The drawing under review shows one solid part. Ordinate dimensions are in mm from its lowest x, y, z. A direction names the side the tool comes from. Coordinates: 2 decimals unless noted, no trailing zeros. Loops run counter-clockwise (first coordinate to the right, second up) from the corner with the lowest first, then second, coordinate; pieces in that order, holes last. Notation, with made-up numbers: (-22, 76) -> (13, 76) arc R38 ccw to (13, 114) -> close; hole circle Ø8 at (21.5, 3). An arc over 180 degrees is marked (long way). Use a Markdown table: item, result.
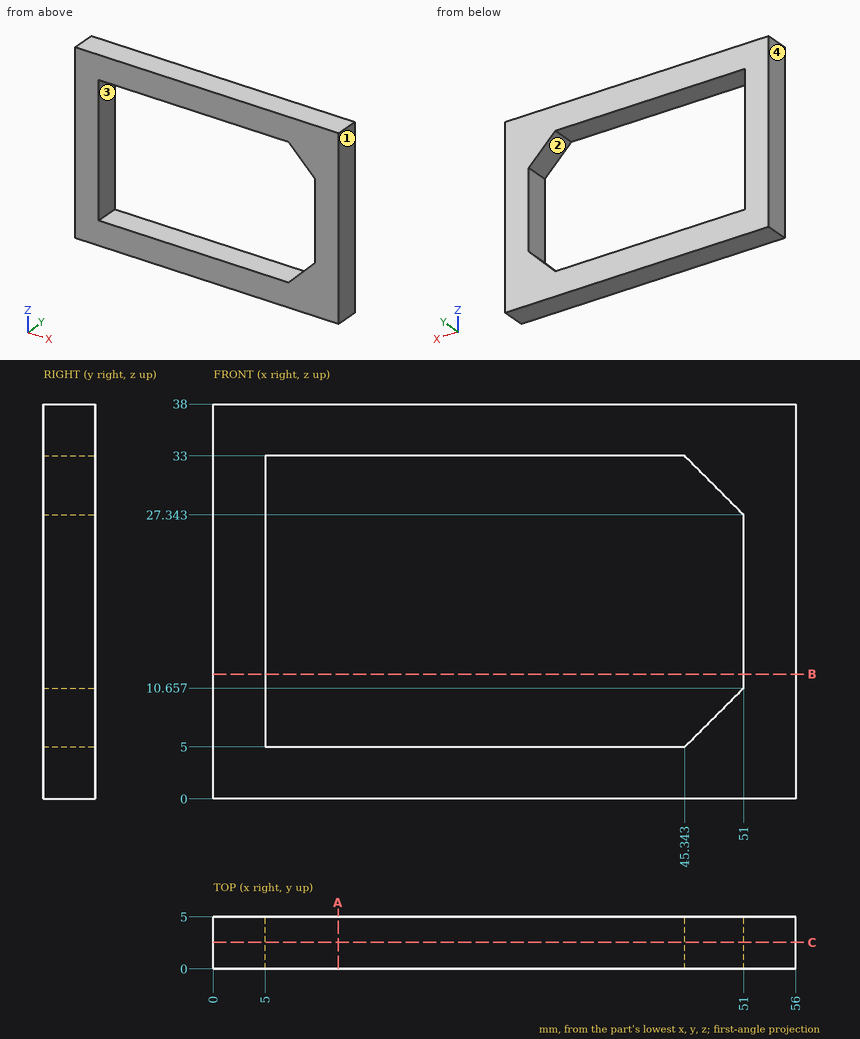
(1) Take a section at A-A on x = 12. Write out the cut boundary in (y, z).
Found:
| item | result |
|---|---|
| outline | (0, 0) -> (5, 0) -> (5, 5) -> (0, 5) -> close; (0, 33) -> (5, 33) -> (5, 38) -> (0, 38) -> close |
(2) For the marked faces 3 and 4, list the 3-axis set-ups (+Z, -Z, +X, -X, +Y, -Y) from which the entire face can be reached by the end or side of a thin tool; tool diameter is ignored.
Found:
| item | result |
|---|---|
| face 3 | +Y, -Y |
| face 4 | +Z, -Z, -X, +Y, -Y |
(3) Mouldability with a two-part tool opening along Z and no side actions: class the marked faces 1 and 2 as pulls with the +Z half, pulls with the -Z half, needs draft (parallel to the pull), parting line crosses it, or undercut.
Found:
| item | result |
|---|---|
| face 1 | needs draft |
| face 2 | undercut |
(4) Take a section at B-B on z = 12. Write out the cut boundary in (x, y).
Found:
| item | result |
|---|---|
| outline | (0, 0) -> (5, 0) -> (5, 5) -> (0, 5) -> close; (51, 0) -> (56, 0) -> (56, 5) -> (51, 5) -> close |
(5) For pin 1 Ø1.5 at (x, z) = (43, 6.5) entering from +Y, flat-tipped, find the tip position at first contact; note if it passes through.
Found:
| item | result |
|---|---|
| pin 1 | passes through |
(6) Take a section at C-C on y = 2.55. Write out the cut boundary in (x, z).
Found:
| item | result |
|---|---|
| outline | (0, 0) -> (56, 0) -> (56, 38) -> (0, 38) -> close; hole (5, 5) -> (45.34, 5) -> (51, 10.66) -> (51, 27.34) -> (45.34, 33) -> (5, 33) -> close |
(7) For line 1 along X through (y, z) = (1.2, 24); line 2 along Z through (x, y) = (7, 2.5); line 3 along X through (y, z) = (2.05, 10.5) (1 decimal), list the stretches that pass through material, from the lowest coordinate up.
Found:
| item | result |
|---|---|
| line 1 | x = 0 to 5, 51 to 56 |
| line 2 | z = 0 to 5, 33 to 38 |
| line 3 | x = 0 to 5, 50.8 to 56 |
